Design review of the part built by this model. Coordinates are the model's own, in mm. A direction names the side the tool comes from. Give positions to 0.01 mm unless a question says otherwise; leave off trailing zeros. Loops run counter-clockwise (first coordinate to the right, second up) from the corner with the lowest first, then second, coordinate; pieces in that order, holes last. Notation, with made-up numbers: M -7.75,50.5 L 43.25,50.5 A20 cw 43.25,81.5 Z; hole C 66,-35 d10. An arc over 180 degrees is marked long. Use CSV: the item, a comma, the result in double quotes.
from build123d import *

# Parameters (mm, degrees)
F0_W     = 102
F0_H     = 84
F0_R     = 2.25
F0_W_2   = 78
F0_H_2   = 51
F1_DEPTH = 15
F3_DEPTH = 4
F4_W     = 12
F4_H     = 44
F4_W_2   = 60
F4_H_2   = 13
F5_DEPTH = 15.001
F6_W     = 102
F6_H     = 84
F7_DEPTH = 8
F8_R     = 5


with BuildPart() as f1:
    # F0 (on Top) → F1 (new body)
    with BuildSketch(Plane.XY):
        with Locations((0, -1.5)):
            Rectangle(F0_W, F0_H)
        with Locations((-44, -32.5)):
            Circle(F0_R, mode=Mode.SUBTRACT)
        with Locations((44, -32.5)):
            Circle(F0_R, mode=Mode.SUBTRACT)
        with Locations((-44, 32.5)):
            Circle(F0_R, mode=Mode.SUBTRACT)
        Rectangle(F0_W_2, F0_H_2, mode=Mode.SUBTRACT)
        with Locations((44, 32.5)):
            Circle(F0_R, mode=Mode.SUBTRACT)
    extrude(amount=F1_DEPTH)

    # F2 (on face) → F3 (cut)
    with BuildSketch(Plane(origin=(0, 0, 0), x_dir=(1, 0, 0), z_dir=(0, 0, -1))):
        Polygon((-41.075, 30.8112504626), (-41.075, 34.1887495374), (-44, 35.8774990748), (-46.925, 34.1887495374), (-46.925, 30.8112504626), (-44, 29.1225009252), align=None)
        Polygon((41.075, 34.1887495374), (41.075, 30.8112504626), (44, 29.1225009252), (46.925, 30.8112504626), (46.925, 34.1887495374), (44, 35.8774990748), align=None)
        Polygon((41.075, -30.8112504626), (41.075, -34.1887495374), (44, -35.8774990748), (46.925, -34.1887495374), (46.925, -30.8112504626), (44, -29.1225009252), align=None)
        Polygon((-41.075, -34.1887495374), (-41.075, -30.8112504626), (-44, -29.1225009252), (-46.925, -30.8112504626), (-46.925, -34.1887495374), (-44, -35.8774990748), align=None)
    extrude(amount=-F3_DEPTH, mode=Mode.SUBTRACT)

    # F4 (on face) → F5 (cut, through all)
    with BuildSketch(Plane.XY.offset(15)):
        with Locations((45, 3.5)):
            Rectangle(F4_W, F4_H)
        with Locations((1, -32)):
            Rectangle(F4_W_2, F4_H_2)
    extrude(amount=-F5_DEPTH, mode=Mode.SUBTRACT)

    # F6 (on face) → F7 (cut)
    with BuildSketch(Plane.XY.offset(15)):
        with Locations((0, -1.5)):
            Rectangle(F6_W, F6_H)
    extrude(amount=-F7_DEPTH, mode=Mode.SUBTRACT)

    # F8
    f8_edges = [f1.edges().sort_by_distance(p)[0] for p in [
        (-51, 40.5, 3.5),
        (51, 40.5, 3.5),
        (-51, -43.5, 3.5),
        (51, -43.5, 3.5),
        (51, 25.5, 3.5),
        (51, -18.5, 3.5),
        (39, -18.5, 3.5),
        (31, -25.5, 3.5),
        (-29, -25.5, 3.5),
    ]]
    fillet(f8_edges, radius=F8_R)


solid = f1.part
(1) We need section C-C on y = -32.5. State the section outline as (x, z) points (3 decimals).
A:
outline,"M -51,0 L -46.925,0 L -46.925,4 L -46.25,4 L -46.25,7 L -51,7 Z; M -41.75,4 L -41.075,4 L -41.075,0 L -29,0 L -29,7 L -41.75,7 Z; M 31,0 L 41.075,0 L 41.075,4 L 41.75,4 L 41.75,7 L 31,7 Z; M 46.25,4 L 46.925,4 L 46.925,0 L 51,0 L 51,7 L 46.25,7 Z"
(2) We need section B-B on y = -20.5. State the section outline as (x, z) points, then the cut area to 3 significant figures.
A:
outline,"M -51,0 L -39,0 L -39,7 L -51,7 Z; M 40,0 L 50,0 L 50,7 L 40,7 Z"
area,"154 mm²"
(3) Wall thickness on line 1 along X through (y, z) = (32.5, 6.25); line 2 along X through (y, z) = (-32.5, 6.2); line 3 along Y through (x, z) = (44, 6): over which ranges is each line inside the solid? List them lowest first. Write a range as [from, to].
A:
line 1,"[-51, -46.25], [-41.75, 41.75], [46.25, 51]"
line 2,"[-51, -46.25], [-41.75, -29], [31, 41.75], [46.25, 51]"
line 3,"[-43.5, -34.75], [-30.25, -18.5], [25.5, 30.25], [34.75, 40.5]"
(4) The part is to be moulded in two halves that separate along X. For faces 4 (the flat face through (-42.517, 29.979, 1.972)), 5 (the flat face through (-51, -2, 3)), 6 (the flat face through (51, 33, 3)), say which applies: released by +X, released by -X, zero draft, split by the parting line, or undercut.
A:
face 4,"undercut"
face 5,"released by -X"
face 6,"released by +X"
(5) We need section D-D on y = 32.5. State the section outline as (x, z) points (3 decimals), then the cut area to 3 significant figures.
A:
outline,"M -51,0 L -46.925,0 L -46.925,4 L -46.25,4 L -46.25,7 L -51,7 Z; M -41.75,4 L -41.075,4 L -41.075,0 L 41.075,0 L 41.075,4 L 41.75,4 L 41.75,7 L -41.75,7 Z; M 46.25,4 L 46.925,4 L 46.925,0 L 51,0 L 51,7 L 46.25,7 Z"
area,"640 mm²"
(6) Clearance check with flat-ended pins moving along their axes: P1, Ø7, axis at x = 44, y = -32.5, coming from the -Z side; P2, Ø1.8, axis at x = -43.5, y = 31, coming from the -Z side. State where each tip first meets the part, or that it passes through.
A:
P1,"z = 0"
P2,"z = 4"
(7) We need section A-A on x = -1. State the section outline as (y, z) points.
A:
outline,"M -43.5,0 L -38.5,0 L -38.5,7 L -43.5,7 Z; M 25.5,0 L 40.5,0 L 40.5,7 L 25.5,7 Z"
(8) Machinability: for faces 1 (the flat face through (-44, -35, 4)), 2 (the cylindrical face through (49.5, -42.07, 3.55)), 3 (the flat face through (37, -25.5, 3)), which of the approach directions +Z, -Z, +X, -X, +Y, -Y give a long, thin tool a straight path to every point of the face, cutting with its end or side? Answer none if there is none.
A:
face 1,"-Z"
face 2,"+Z, -Z, +X, -Y"
face 3,"+Z, -Z"
